Study the drawing (mm; zero at the part's minimum x, y, z) and answer. A direction names the side the tool comes from. Coordinates: 2 decimals unless noted, no trailing zeros. Loops run counter-clockwise (first coordinate to the right, second up) from the corner with the lowest first, then second, coordinate; pieces in that order, holes last. Notation, with made-up numbers: (70, 34.25) - (79, 34.25) arc R29 cw to (79, 62.25) - close; hole circle Ø8 at (78.25, -1.5). An arc over 180 degrees is marked (long way). Use one line per item in the form item = value.
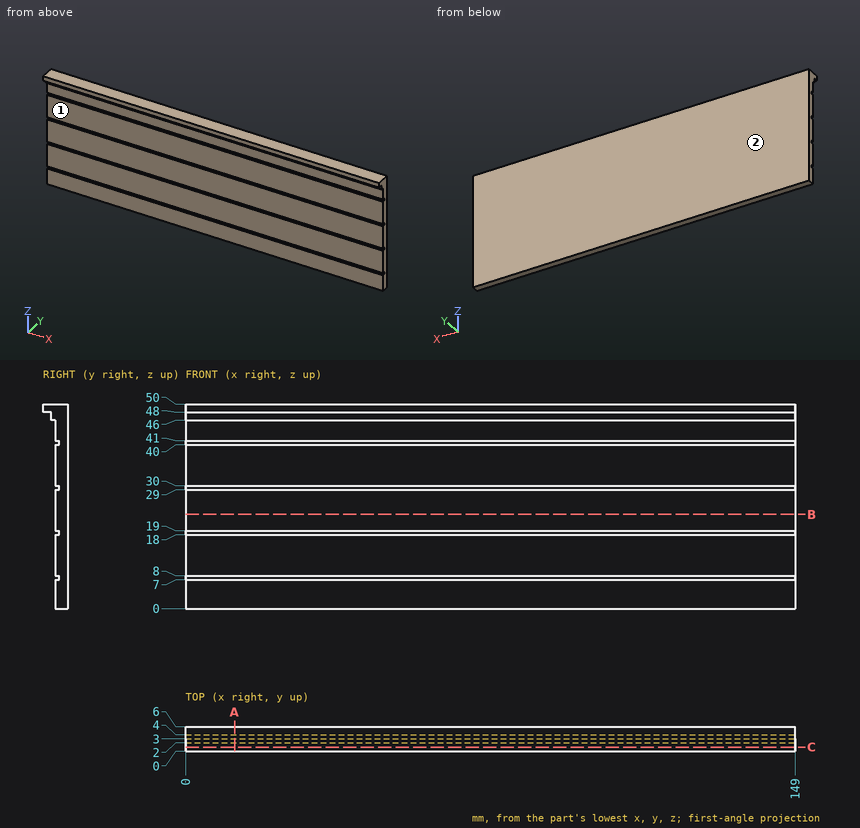
Item 1: Find the intervals of material crossed by L1, parallel to Z at x = 135, y = 3.4; L2, parallel to Y at x = 118, z = 19.5; L3, parallel to Z at x = 33, y = 1.6, in increasing order.
Results below:
L1 = 0 to 7, 8 to 18, 19 to 29, 30 to 40, 41 to 50
L2 = 3 to 6
L3 = 48 to 50
Item 2: The part is cut by section C-C on y = 0.95. Give the vertices of the cut face in (x, z), plus the area to 3 significant figures.
Results below:
outline = (0, 48) - (149, 48) - (149, 50) - (0, 50) - close
area = 298 mm²
Item 3: The part is cut by section A-A on x = 12. Give the vertices of the cut face in (y, z).
Results below:
outline = (0, 48) - (2, 48) - (2, 46) - (3, 46) - (3, 41) - (4, 41) - (4, 40) - (3, 40) - (3, 30) - (4, 30) - (4, 29) - (3, 29) - (3, 19) - (4, 19) - (4, 18) - (3, 18) - (3, 8) - (4, 8) - (4, 7) - (3, 7) - (3, 0) - (6, 0) - (6, 50) - (0, 50) - close
Item 4: The part is cut by section B-B on z = 23. Give the vertices of the cut face in (x, y), plus the area to 3 significant figures.
Results below:
outline = (0, 3) - (149, 3) - (149, 6) - (0, 6) - close
area = 447 mm²
Item 5: Each of these flat-tipped pins is pushed along its axis until it touches: P1, Ø0.6, axis at x = 53, z = 46.5, coming from the -Y side; P2, Ø10, axis at x = 77.5, z = 25.5, coming from the -Y side; P3, Ø0.5, axis at x = 87.5, z = 29.5, coming from the -Y side. Where does it stop, or does it pass through?
Results below:
P1 = 2
P2 = 3
P3 = 4
Item 6: Which of the six approach directions +Z, -Z, +X, -X, +Y, -Y give full straight-line access (tool end or side, diameter ignored) to the marked faces 1 and 2?
Results below:
face_1 = -Z, +X, -X, -Y
face_2 = +Z, -Z, +X, -X, +Y
